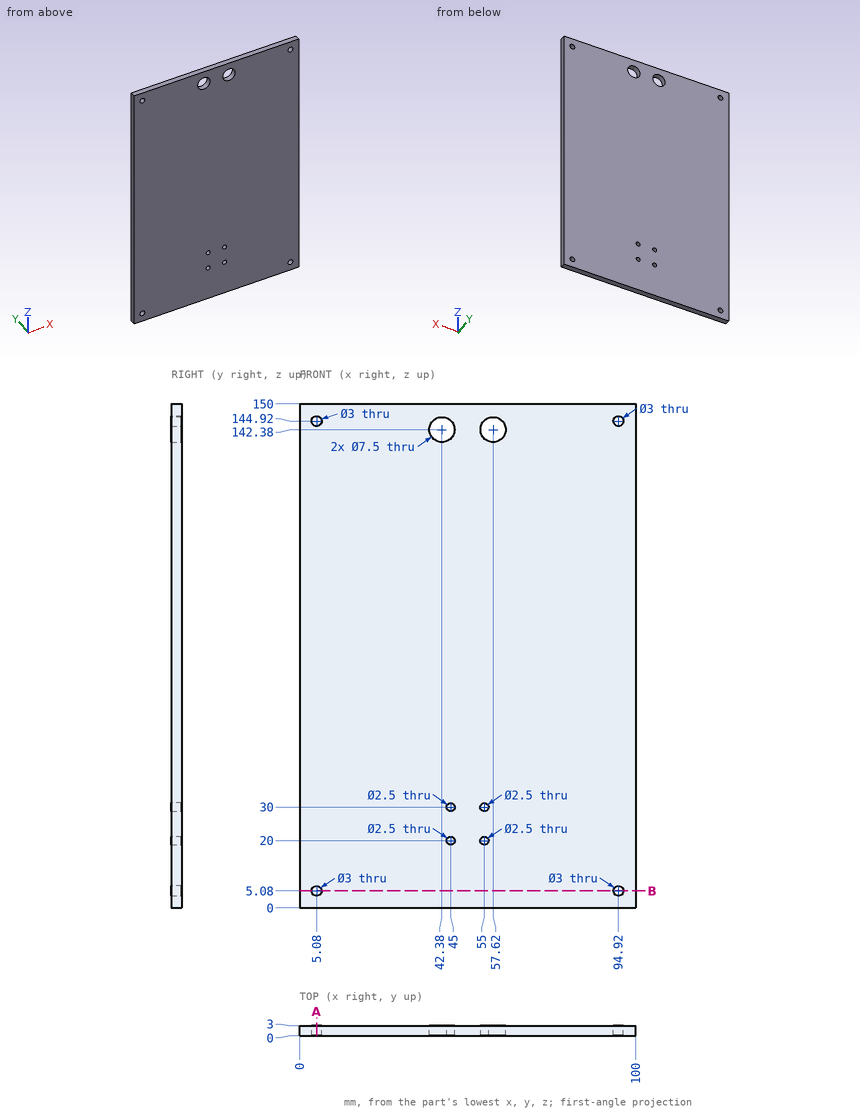
Can you work these out from the drawing? Everything is in mm from the part's minimum corner. Round coordinates to 2 decimals unless told otherwise and drop trailing zeros. Order: outer loops, then holes, each group sorted by start corner. A loop starts at its lowest first (then second) coordinate and runs counter-clockwise, first axis right, second up. Notation, with made-up numbers: (21, 26) -> (75, 26) arc R37 cw to (75, 62) -> close; hole circle Ø11 at (35.25, 77.25). An arc over 180 degrees is marked (long way). Use CSV: the item, a comma, the result in double quotes.
1. I want a section at A-A on x = 5.08. List the corners of the cut face in (y, z) for me, and give its area (3 significant figures).
Recorded:
outline,"(0, 0) -> (3, 0) -> (3, 3.58) -> (0, 3.58) -> close; (0, 6.58) -> (3, 6.58) -> (3, 143.42) -> (0, 143.42) -> close; (0, 146.42) -> (3, 146.42) -> (3, 150) -> (0, 150) -> close"
area,"432 mm2"
2. I need wall thicknesses on line 1 along X through (y, z) = (2.35, 20); line 2 along X through (y, z) = (2.15, 142.38); line 3 along Z through (x, y) = (94.92, 1.8). Which ranges of each line are inside material? Lowest first, please.
Recorded:
line 1,"x = 0 to 43.75, 46.25 to 53.75, 56.25 to 100"
line 2,"x = 0 to 38.63, 46.13 to 53.87, 61.37 to 100"
line 3,"z = 0 to 3.58, 6.58 to 143.42, 146.42 to 150"
3. I want a section at B-B on z = 5.08. List the corners of the cut face in (x, y) for me, and give its area (3 significant figures).
Recorded:
outline,"(0, 0) -> (3.58, 0) -> (3.58, 3) -> (0, 3) -> close; (6.58, 0) -> (93.42, 0) -> (93.42, 3) -> (6.58, 3) -> close; (96.42, 0) -> (100, 0) -> (100, 3) -> (96.42, 3) -> close"
area,"282 mm2"
